CAD build for the part. Positions are in the model's coordinates, mm. A direction names the side the tool comes from. Round coordinates to 2 decimals unless told otherwise and drop trailing zeros. Order: outer loops, then holes, each group sorted by start corner. A loop starts at its lowest first (then second) coordinate and runs counter-clockwise, first axis right, second up. Notation, with made-up numbers: M 6,70.5 L 14,70.5 A25 cw 14,107.5 Z; hole C -6.75,13.25 d3. An arc over 180 degrees is marked long. Answer as CSV lines item,"result". Start each with the question number.
Autodesk Inventor part; units mm, degrees
ref_plane "YZ Plane" through (0, 0, 0) normal (1, 0, 0) x (0, 1, 0)
ref_plane "XZ Plane" through (0, 0, 0) normal (0, 1, 0) x (-1, 0, 0)
ref_plane "XY Plane" through (0, 0, 0) normal (0, 0, 1) x (1, 0, 0)
sketch "Skizze1" plane through (0, 0, 0) normal (0, 0, 1) x (1, 0, 0)
  line L0 (0, 0) -> (40, 0)
  line L1 (5, 5) -> (5, 50)
  line L2 (5, 50) -> (0, 50)
  line L3 (0, 50) -> (0, 0)
  line L4 (5, 5) -> (40, 5)
  line L5 (40, 5) -> (40, 0)
  line L6 (-8, 0) -> (48, 0)
  line L7 (0, -10) -> (0, 60)
  dimension "d0" = 50
  dimension "d3" = 40
  dimension "d4" = 5
extrude "Extrusion1" add sketch "Skizze1" along normal blind 40
sketch "Skizze2" plane through (0, 0, 0) normal (-1, 0, 0) x (0, 0, 1)
  line L0 (0, 50) -> (40, 50)
  line L1 (0, 0) -> (40, 0)
  line L2 (20, 50) -> (20, 0)
  point P0 (20, 27)
  dimension "d7" = 27
hole "Bohrung1" at (0, 27, 20) direction (1, 0, 0) diameter 22 end through all
sketch "Skizze4" plane through (0, 0, 0) normal (0, -1, 0) x (1, 0, 0)
  line L0 (40, 40) -> (0, 40)
  line L1 (0, 0) -> (0, 40)
  line L2 (0, 0) -> (40, 0)
  line L3 (40, 0) -> (40, 40)
  line L4 (28, 40) -> (28, 0)
  line L5 (0, 20) -> (40, 20)
  point P0 (28, 29)
  point P1 (28, 11)
  dimension "d24" = 12
  dimension "d25" = 18
hole "Bohrung3" at (28, 0, 29) at (28, 0, 11) direction (0, 1, 0) diameter 4.5 end through all
hole "Bohrung4" at (28, 5, 29) direction (0, -1, 0) diameter 4.5 end through all countersink diameter 9.2 countersink angle 90
hole "Bohrung5" at (28, 5, 11) direction (0, -1, 0) diameter 4.5 end through all countersink diameter 9.2 countersink angle 90
chamfer "Fase1" distance 10 angle 45 2 edges at (40, 2.5, 0) (40, 2.5, 40)
sketch "Skizze6" plane through (5, 5, 0) normal (1, 0, 0) x (0, 0, -1)
  circle A0 centre (-20, 22) radius 11
  line L0 (0, 45) -> (-40, 45)
  line L1 (-20, 22) -> (-5.2877, 22)
  line L2 (0, -15.2) -> (0, 56.2)
  line L3 (8, -5) -> (-48, -5)
  line L4 (-20, 22) -> (-20, 10.2851)
  line L5 (-35.5, 37.5) -> (-4.5, 37.5)
  line L6 (-4.5, 37.5) -> (-4.5, 6.5)
  line L7 (-4.5, 6.5) -> (-35.5, 6.5)
  line L8 (-35.5, 6.5) -> (-35.5, 37.5)
  point P0 (0, -5)
  dimension "d54" = 31
hole "Bohrung6" at (5, 42.5, 35.5) at (5, 42.5, 4.5) at (5, 11.5, 4.5) at (5, 11.5, 35.5) direction (-1, 0, 0) diameter 3.4 end through all
chamfer "Fase2" distance 5 angle 45 2 edges at (2.5, 50, 40) (2.5, 50, 0)
properties part number "13_0204_058"
Q1. Band-saw the part on C-C, the plane x = 28. Write the cut outline in (y, z).
Q2. Band-saw the part on B-B, the plane z = 20. Write the cut outline in (x, y).
Q3. Probe line 1 along Z through (x, y) = (3.8, 11.5); line 2 along Z through (x, y) = (28, 1.2); line 3 along Y through (x, z) = (3.75, 4.5). List the from-to ranges inside material, lowest first. Write a range as from..to.
Q4. Band-saw the part on D-D, the plane y = 27. Write the cut outline in (x, z).
Q5. Band-saw the part on A-A, the plane y = 11.5. Write the cut outline in (x, z).
Q6. Tool access for faces 1 (the flat face through (35, 3, 5)), 2 (the flat face through (22, 5, 20)): list every direction of +Z, -Z, +X, -X, +Y, -Y with a clear straight run to the whole face (end or side of a thin tool).
Q7. Drop flat-ended pins along their axis: P1, Ø10, axis at y = 20, z = 22, coming from the +X side; P2, Ø2, axis at x = 30.5, z = 33.5, coming from the +Y side. Give the stop position or say it passes through.
Q8. Mould opens along Y. For faces 3 (the conical face through (25.66, 2.797, 10.48)), 4 (the cylindrical face through (2.5, 13, 3.7)), 5 (the flat face through (4, 19, 40)) say: +Y half, -Y half, draft (parallel to the pull), parting line (faces both ways), or undercut.
Answer:
1,outline,"M 0,0 L 5,0 L 5,6.4 L 2.65,8.75 L 0,8.75 Z; M 0,13.25 L 2.65,13.25 L 5,15.6 L 5,24.4 L 2.65,26.75 L 0,26.75 Z; M 0,31.25 L 2.65,31.25 L 5,33.6 L 5,40 L 0,40 Z"
2,outline,"M 0,0 L 40,0 L 40,5 L 5,5 L 5,16 L 0,16 Z; M 0,38 L 5,38 L 5,50 L 0,50 Z"
3,line 1,"z = 0..2.8, 6.2..33.8, 37.2..40"
3,line 2,"z = 0..8.75, 13.25..26.75, 31.25..40"
3,line 3,"y = 0..9.8, 13.2..40.8, 44.2..49.5"
4,outline,"M 0,0 L 5,0 L 5,9 L 0,9 Z; M 0,31 L 5,31 L 5,40 L 0,40 Z"
5,outline,"M 0,0 L 5,0 L 5,2.8 L 0,2.8 Z; M 0,6.2 L 5,6.2 L 5,33.8 L 0,33.8 Z; M 0,37.2 L 5,37.2 L 5,40 L 0,40 Z"
6,face 1,"-Z, +X, +Y, -Y"
6,face 2,"+Z, -Z, +X, +Y"
7,P1,"stops at x = 5"
7,P2,"stops at y = 5"
8,face 3,"+Y half"
8,face 4,"undercut"
8,face 5,"draft"
